Design review of the part shown in the three views and the two pictorial views. Dimensions are in mm from the part's minimum x, y and z. Coordinates: 2 decimals unless noted, no trailing zeros. Write each loop counter-clockwise with the first axis right and the second up, starting at its lowest first coordinate (ties: lowest second). Pieces come first, ordered by that corner, then holes. Notation, with made-up numbers: (56.25, 51) - (113.25, 51) arc R7 ccw to (113.25, 55) - close; hole circle Ø11 at (-29.75, 19.5). An arc over 180 degrees is marked (long way). Return JSON: item names as keys, results as strings. Group by question number.
(1) For pin 1 Ø5 at (x, y) = (9, 28.5) entering from -Z (1 decimal); pin 2 Ø12 at (x, y) = (66.5, 20.5) entering from -Z; pin 3 Ø1.5 at (x, y) = (48.5, 37) entering from -Z (1 decimal); pin 4 Ø5 at (x, y) = (12.7, 42.33) entering from +Z, all flat-tipped, find the tip position at first contact; note any pin that passes through.
(2) We need section B-B on y = 4. State the section outline as (x, z) points, then the cut area to 3 significant figures.
(3) We need section A-A on z = 20.5. Give the number of separate pieces and of enclosed holes in the cut face, then the cut area to 3 significant figures.
(4) To check wall thickness, follow L1, parallel to Y at x = 64, z = 29; L2, parallel to Y at x = 19, z = 12; L3, parallel to Y at x = 63, z = 27. State the ranges of each line that lie inside material, in increasing order. Write a range as from..to.
(5) We need section D-D on z = 4. State the section outline as (x, y) points.
(6) Draft analysis for pull direction X (two halves, no side actions). For the marked faces 1, 2, 3 and 4, state which applies: released by +X, released by -X, zero draft, split by the parting line, or undercut.
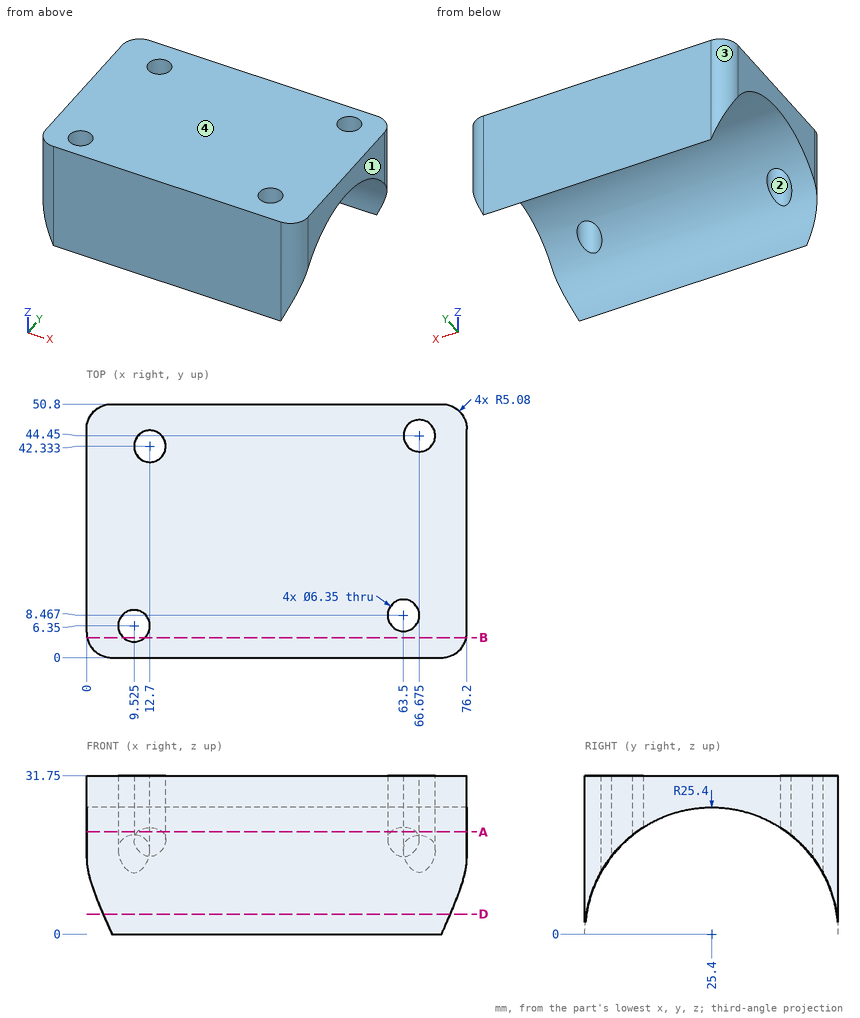
Ans:
{
 "1": {"pin 1": "z = 24.8", "pin 2": "z = 22.94", "pin 3": "z = 22.2", "pin 4": "through"},
 "2": {"outline": "(0.12, 13.68) - (7.39, 13.68) - (7.39, 31.75) - (0.12, 31.75) - close; (11.66, 13.68) - (76.08, 13.68) - (76.08, 31.75) - (11.66, 31.75) - close", "area": "1,300 mm²"},
 "3": {"separate pieces": "2", "enclosed holes": "2", "area": "1,450 mm²"},
 "4": {"L1": "0..5.33, 11.6..42.74, 46.16..50.8", "L2": "0..3.01, 47.79..50.8", "L3": "0..5.33, 11.6..50.8"},
 "5": {"outline": "(3.31, 0.32) arc R5.08 ccw to (5.08, 0) - (71.12, 0) arc R5.08 ccw to (72.89, 0.32) - close; (3.31, 50.48) - (72.89, 50.48) arc R5.08 ccw to (71.12, 50.8) - (5.08, 50.8) arc R5.08 ccw to start"},
 "6": {"face 1": "released by +X", "face 2": "undercut", "face 3": "released by -X", "face 4": "zero draft"}
}
